from build123d import *

# Parameters (mm, degrees)
ESQUISSE1_W             = 60
ESQUISSE1_H             = 24
ESQUISSE1_R             = 2.5
BOSS_EXTRU_1_DEPTH      = 2
BOSS_EXTRU_2_DEPTH      = 2
ESQUISSE3_W             = 60
ESQUISSE3_H             = 4.5
BOSS_EXTRU_3_DEPTH      = 20
ESQUISSE5_W             = 5
ESQUISSE5_H             = 5
ENL_V_MAT_EXTRU_2_DEPTH = 8
ESQUISSE6_W             = 5
ESQUISSE6_H             = 5
ENL_V_MAT_EXTRU_3_DEPTH = 8


with BuildPart() as part:
    # Esquisse1 → Boss.-Extru.1 (new body)
    with BuildSketch(Plane(origin=(0, 0, 0), x_dir=(1, 0, 0), z_dir=(0, 1, 0))):
        with Locations((30, 0)):
            Rectangle(ESQUISSE1_W, ESQUISSE1_H)
        with Locations((10, 0)):
            Circle(ESQUISSE1_R, mode=Mode.SUBTRACT)
    extrude(amount=BOSS_EXTRU_1_DEPTH)

    # Esquisse2 → Boss.-Extru.2 (add)
    with BuildSketch(Plane(origin=(0, 2, 0), x_dir=(1, 0, 0), z_dir=(0, 1, 0))):
        Polygon((60, 12), (33, 12), (33, 10), (58, 10), (58, -10), (33, -10), (33, -12), (60, -12), align=None)
    extrude(amount=BOSS_EXTRU_2_DEPTH)

    # Esquisse3 → Boss.-Extru.3 (add)
    with BuildSketch(Plane.XZ):
        with Locations((30, 9.75)):
            Rectangle(ESQUISSE3_W, ESQUISSE3_H)
        with Locations((30, -9.75)):
            Rectangle(ESQUISSE3_W, ESQUISSE3_H)
    extrude(amount=BOSS_EXTRU_3_DEPTH)

    # Esquisse5 → Enlèv. mat.-Extru.2 (cut)
    with BuildSketch(Plane.XY.offset(12)):
        with Locations((55, -0.5)):
            Rectangle(ESQUISSE5_W, ESQUISSE5_H)
    extrude(amount=-ENL_V_MAT_EXTRU_2_DEPTH, mode=Mode.SUBTRACT)

    # Esquisse6 → Enlèv. mat.-Extru.3 (cut)
    with BuildSketch(Plane(origin=(0, 0, -12), x_dir=(-1, 0, 0), z_dir=(0, 0, -1))):
        with Locations((-43, -0.5)):
            Rectangle(ESQUISSE6_W, ESQUISSE6_H)
    extrude(amount=-ENL_V_MAT_EXTRU_3_DEPTH, mode=Mode.SUBTRACT)


solid = part.part
Verification items for the finished model (mm, model axes). A direction names the side the tool comes from. Round coordinates to 2 decimals unless told otherwise and drop trailing zeros. Order: outer loops, then holes, each group sorted by start corner. A loop starts at its lowest first (then second) coordinate and runs counter-clockwise, first axis right, second up.
1. Go/stop test with flat-tipped pins: P1, Ø8, axis at x = 22, z = -4.5, coming from the +Y side; P2, Ø2, axis at y = 3.5, z = 2, coming from the -X side; P3, Ø0.6, axis at y = 3, z = -11.5, coming from the -X side. Record where each tip stops, or that it passes through.
Final values:
P1: stops at y = 2
P2: stops at x = 58
P3: stops at x = 33
2. Release check for a two-part mould opening along Y. For faces 1 (the flat face through (55, -3, 10)), 2 (the flat face through (55, 1, 4)), 3 (the flat face through (43, 2, -11)), 4 (the flat face through (58.4, 4, 1.7)) record: +Y half, -Y half, draft (parallel to the pull), parting line (faces both ways), or undercut.
Final values:
face 1: undercut
face 2: draft
face 3: undercut
face 4: +Y half
3. Thickness scan on L1, parallel to Z at x = 35.5, y = -2.75; L2, parallel to Z at x = 10, y = 1.45; L3, parallel to X at y = 0.6, z = 0. Record the ranges inside material, lowest first.
Final values:
L1: z = -12 to -7.5, 7.5 to 12
L2: z = -12 to -2.5, 2.5 to 12
L3: x = 0 to 7.5, 12.5 to 60
4. Section check D-D on y = -1. Record the cut outline in (x, z).
Final values:
outline: (0, -12) - (40.5, -12) - (40.5, -7.5) - (0, -7.5) - close; (0, 7.5) - (52.5, 7.5) - (52.5, 12) - (0, 12) - close; (45.5, -12) - (60, -12) - (60, -7.5) - (45.5, -7.5) - close; (57.5, 7.5) - (60, 7.5) - (60, 12) - (57.5, 12) - close
5. Access from +Z, -Z, +X, -X, +Y, -Y to the whole of each face (thin tool, end or side, straight path). Record for faces 5 (the flat face through (45.5, 0, -9)), 6 (the flat face through (33, 3, 11)), 7 (the flat face through (30, -10, 7.5)).
Final values:
face 5: -Z
face 6: +Z, -Z, -X, +Y
face 7: +X, -X, -Y
6. Section check A-A on y = -18. Record the cut outline in (x, z).
Final values:
outline: (0, -12) - (60, -12) - (60, -7.5) - (0, -7.5) - close; (0, 7.5) - (60, 7.5) - (60, 12) - (0, 12) - close
7. Section check B-B on x = 10. Record the cut outline in (y, z), then the cut area to 3 significant figures.
Final values:
outline: (-20, -12) - (2, -12) - (2, -2.5) - (0, -2.5) - (0, -7.5) - (-20, -7.5) - close; (-20, 7.5) - (0, 7.5) - (0, 2.5) - (2, 2.5) - (2, 12) - (-20, 12) - close
area: 218 mm2
8. Section check C-C on z = 0. Record the cut outline in (x, y), then the cut area to 3 significant figures.
Final values:
outline: (0, 0) - (7.5, 0) - (7.5, 2) - (0, 2) - close; (12.5, 0) - (60, 0) - (60, 4) - (58, 4) - (58, 2) - (12.5, 2) - close
area: 114 mm2
